Build history of the part. All positions in model axes, mm. A direction names the side the tool comes from. Give positions to 0.01 mm unless a question says otherwise; leave off trailing zeros. Loops run counter-clockwise (first coordinate to the right, second up) from the corner with the lowest first, then second, coordinate; pieces in that order, holes last. Notation, with made-up numbers: M 66.25,27 L 97.25,27 A9 cw 97.25,31 Z; hole C 34.25,-17 d6. An arc over 180 degrees is marked long. Answer in a Markdown table with one row per item. Add a question column.
```python
from build123d import *

# Parameters (mm, degrees)
F0_W           = 116.2
F0_H           = 46
F0_W_2         = 91.2
F0_H_2         = 37
F1_DEPTH       = 14
F3_DEPTH       = 116.201
F4_T           = -3.85
F5_W           = 91.2
F5_H           = 37
F6_DEPTH       = 14.001
F7_R           = 2.8
F7_R_2         = 2.85
F10_DEPTH      = 25
F11_R          = 1.225
F12_DEPTH      = 10
F14_R          = 1.1
F15_DEPTH      = 3
F15_DEPTH_BACK = 1.955065151
F16_R          = 1.225
F16_R_2        = 2.8
F17_DEPTH      = 3.7


with BuildPart() as f1:
    # F0 (on Top) → F1 (new body)
    with BuildSketch(Plane.XY):
        Rectangle(F0_W, F0_H)
        Rectangle(F0_W_2, F0_H_2, mode=Mode.SUBTRACT)
        Rectangle(F0_W_2, F0_H_2)
    extrude(amount=F1_DEPTH)

    # F2 (on face) → F3 (cut, through all)
    with BuildSketch(Plane.YZ.offset(58.1)):
        Polygon((23, 14), (23, 8.5), (26.9685778767, 8.2080848515), (26.9685778767, 18.4987988323), (-26.2719616294, 18.4987988323), (-26.2719616294, 8.5), (-23, 8.5), (-23, 14), (0, 14), align=None)
        with BuildLine():
            ThreePointArc((-23, 8.5), (-11.8242335904, 12.6058859234), (0, 14))
            Line((0, 14), (-23, 14))
            Line((-23, 14), (-23, 8.5))
        make_face()
        with BuildLine():
            ThreePointArc((0, 14), (11.8242335904, 12.6058859234), (23, 8.5))
            Line((23, 8.5), (23, 14))
            Line((23, 14), (0, 14))
        make_face()
    extrude(amount=-F3_DEPTH, mode=Mode.SUBTRACT)

    # F4
    f4_openings = [f1.faces().sort_by_distance(p)[0] for p in [
        (0, 0, 0),
    ]]
    offset(amount=F4_T, openings=f4_openings)

    # F5 (on Top) → F6 (cut, through all)
    with BuildSketch(Plane.XY):
        Rectangle(F5_W, F5_H)
    extrude(amount=F6_DEPTH, mode=Mode.SUBTRACT)

    # F7 (on face) → F8 (join, up to the next surface of F1)
    with BuildSketch(Plane(origin=(0, 0, 0), x_dir=(1, 0, 0), z_dir=(0, 0, -1))):
        with Locations((-49.4, 14.3)):
            Circle(F7_R)
        with Locations((-49.4, -14.3)):
            Circle(F7_R)
        with Locations((52.4, 13.5)):
            Circle(F7_R)
        with Locations((52.4, -13.5)):
            Circle(F7_R_2)
    extrude(until=Until.NEXT, dir=(0, 0, 1))

    # F9 (on face) → F10 (cut)
    with BuildSketch(Plane.YZ.offset(58.1)):
        with BuildLine():
            ThreePointArc((-5.5, 0), (0, -5.5), (5.5, 0))
            Line((5.5, 0), (-5.5, 0))
        make_face()
        with BuildLine():
            Line((-5.5, 0), (5.5, 0))
            ThreePointArc((5.5, 0), (0, 5.5), (-5.5, 0))
        make_face()
    extrude(amount=-F10_DEPTH, mode=Mode.SUBTRACT)

    # F11 (on face) → F12 (cut)
    with BuildSketch(Plane(origin=(0, 0, 0), x_dir=(1, 0, 0), z_dir=(0, 0, -1))):
        with Locations((-49.4, 14.3)):
            Circle(F11_R)
        with Locations((-49.4, -14.3)):
            Circle(F11_R)
        with Locations((52.4, 13.5)):
            Circle(F11_R)
        with Locations((52.4, -13.5)):
            Circle(F11_R)
    extrude(amount=-F12_DEPTH, mode=Mode.SUBTRACT)

    # F14 (on offset) → F15 (join, two sides)
    with BuildSketch(Plane(origin=(0, 0, 8), x_dir=(1, 0, 0), z_dir=(0, 0, -1))) as f15_sk:
        with BuildLine():
            Line((47.0988332987, 11.1403603734), (47.0988332987, 4.8591672747))
            ThreePointArc((47.0988332987, 4.8591672747), (52.8239783636, 7.999763824), (47.0988332987, 11.1403603734))
        make_face()
        with Locations((49.1, 7.999763824)):
            Circle(F14_R, mode=Mode.SUBTRACT)
        with BuildLine():
            ThreePointArc((47.0968177208, -10.9978726761), (52.6833744029, -8.0229183659), (47.0968177208, -5.0479640557))
            Line((47.0968177208, -5.0479640557), (47.0968177208, -10.9978726761))
        make_face()
        with Locations((49.0979844222, -8.0229183659)):
            Circle(F14_R, mode=Mode.SUBTRACT)
    extrude(amount=F15_DEPTH)
    extrude(f15_sk.sketch, amount=-F15_DEPTH_BACK)

    # F16 (on face) → F17 (join)
    with BuildSketch(Plane(origin=(0, 0, 0), x_dir=(1, 0, 0), z_dir=(0, 0, -1))):
        with BuildLine():
            ThreePointArc((54.25, 11.3982150443), (55.2, 13.5), (54.25, 15.6017849557))
            ThreePointArc((54.25, 15.6017849557), (49.6, 13.5), (54.25, 11.3982150443))
        make_face()
        with Locations((52.4, 13.5)):
            Circle(F16_R, mode=Mode.SUBTRACT)
        with BuildLine():
            ThreePointArc((54.25, -15.6679483389), (55.25, -13.5), (54.25, -11.3320516611))
            ThreePointArc((54.25, -11.3320516611), (49.55, -13.5), (54.25, -15.6679483389))
        make_face()
        with Locations((52.4, -13.5)):
            Circle(F16_R, mode=Mode.SUBTRACT)
        with Locations((-49.4, 14.3)):
            Circle(F16_R_2)
        with Locations((-49.4, 14.3)):
            Circle(F16_R, mode=Mode.SUBTRACT)
        with Locations((-49.4, -14.3)):
            Circle(F16_R_2)
        with Locations((-49.4, -14.3)):
            Circle(F16_R, mode=Mode.SUBTRACT)
    extrude(amount=F17_DEPTH)


solid = f1.part
```
(1) Wall check: line 1 (Y direction, x = -49.4, z = -2.5) (3 decimals); line 2 (Y direction, x = -49.4, z = 5.75) (3 decimals); line 3 (Y direction, x = 45, z = 1.5). Give the ranges that are in metal, low to high.
(2) Slice it at B-B, the plane z = 3. Give the cut face in (x, y) (3 decimals), then the cut area to 3 significant figures.
(3) Pull direction X, two halves, no side cores. Call faces 4 (the flat face through (58.1, 0, 7)), 5 (the cylindrical face through (49.12, -8.02, 9.46)), 6 (the flat face through (-1, -23, 4)): +X half, -X half, draft (parallel to the pull), parting line (faces both ways), or undercut.
(4) Tool access for faces 1 (the flat face through (54, -13, -3.7)), 2 (the flat face through (45.6, 0, 11)), 3 (the flat face through (-49, -14, 10)): list every direction of +Z, -Z, +X, -X, +Y, -Y with a clear straight run to the whole face (end or side of a thin tool).
(5) Slice it at A-A, the plane x = -41.5. Give the cut face in (y, z).
(6) Slice it at C-C, the plane z = 12.5. Give the cut face in (x, y), then the cut area to 3 significant figures.
(7) Pin check, flat tips, straight feed: pin 1 (3.5 mm diameter, centred on x = 49.1, y = -8, fed in from +Z); pin 2 (2 mm diameter, centred on x = 52.4, y = -13.5, fed in from -Z); pin 3 (1.3 mm diameter, centred on x = 49.1, y = 8.02, fed in from +Z). Stop position of each tip, or through.
Solution:
| question | item | result |
|---|---|---|
| 1 | line 1 | -17.1 to -15.525, -13.075 to -11.5, 11.5 to 13.075, 15.525 to 17.1 |
| 1 | line 2 | -23 to -19.15, -17.1 to -15.525, -13.075 to -11.5, 11.5 to 13.075, 15.525 to 17.1, 19.15 to 23 |
| 1 | line 3 | -23 to -19.15, 19.15 to 23 |
| 2 | outline | M -58.1,-23 L 58.1,-23 L 58.1,-4.61 L 54.25,-4.61 L 54.25,-11.398 A2.8 ccw long 54.25,-15.602 L 54.25,-19.15 L -54.25,-19.15 L -54.25,19.15 L 54.25,19.15 L 54.25,15.668 A2.85 ccw long 54.25,11.332 L 54.25,4.61 L 58.1,4.61 L 58.1,23 L -58.1,23 Z; C -49.4,-14.3 d5.6; C -49.4,14.3 d5.6; hole C -49.4,-14.3 d2.45; hole C -49.4,14.3 d2.45; hole C 52.4,-13.5 d2.45; hole C 52.4,13.5 d2.45 |
| 2 | area | 1,230 mm^2 |
| 3 | face 4 | +X half |
| 3 | face 5 | undercut |
| 3 | face 6 | draft |
| 4 | face 1 | -Z, +X, -X, +Y, -Y |
| 4 | face 2 | +Z, -Z |
| 4 | face 3 | -Z |
| 5 | outline | M -23,0 L -19.15,0 L -19.15,6.07 A46.99 cw -18.5,6.36 L -18.5,10.51 A50.84 ccw -23,8.5 Z; M 18.5,6.36 A46.99 cw 19.15,6.07 L 19.15,0 L 23,0 L 23,8.5 A50.84 ccw 18.5,10.51 Z |
| 6 | outline | M -58.1,-12.26 L -45.6,-12.26 L -45.6,12.26 L -58.1,12.26 Z; M 45.6,-12.26 L 58.1,-12.26 L 58.1,12.26 L 45.6,12.26 Z |
| 6 | area | 613 mm^2 |
| 7 | pin 1 | z = 13.61 |
| 7 | pin 2 | z = 10 |
| 7 | pin 3 | z = 13.46 |
